```python
from build123d import *

# Parameters (mm, degrees)
F1_DEPTH = 63.5
F0_W     = 25.4
F0_H     = 16.5099985898
F2_DEPTH = 25.4
F3_DEPTH = 8.255


with BuildPart() as f1:
    # F0 (on Front) → F1 (new body, symmetric)
    with BuildSketch(Plane.XZ):
        Polygon((24.7650014102, 9.525), (-41.275, 9.525), (-41.275, -9.525), (41.275, -9.525), (41.275, 9.525), align=None)
    extrude(amount=F1_DEPTH, both=True)

    # F0 (on Front) → F2 (join, symmetric)
    with BuildSketch(Plane.XZ):
        with BuildLine():
            Line((24.7650014102, 27.0002), (24.7650014102, 9.525))
            Line((24.7650014102, 9.525), (41.275, 9.525))
            Line((41.275, 9.525), (41.275, 27.0002))
            ThreePointArc((41.275, 27.0002), (45.9246798487, 38.2255201513), (57.15, 42.8752))
            Line((57.15, 42.8752), (60.325, 42.8752))
            Line((60.325, 42.8752), (60.325, 59.3851985898))
            Line((60.325, 59.3851985898), (57.15, 59.3851985898))
            add(Edge.make_bspline(
                [(56.1071182256, 59.3684024719), (56.4564666589, 59.3745204877), (56.8041138662, 59.3801120386), (57.15, 59.3851985898)],
                knots=[109.340800828, 109.340800828, 109.340800828, 109.340800828, 110.3336758583, 110.3336758583, 110.3336758583, 110.3336758583], degree=3))
            ThreePointArc((56.1071182256, 59.3684024719), (33.8845550392, 49.5281205528), (24.7650014102, 27.0002))
        make_face()
        with Locations((73.025, 51.1301992949)):
            Rectangle(F0_W, F0_H)
    extrude(amount=F2_DEPTH, both=True)

    # F0 (on Front) → F3 (join, symmetric)
    with BuildSketch(Plane.XZ):
        with BuildLine():
            add(Edge.make_bspline(
                [(-41.275, 9.525), (-41.4689933248, 51.6361419003), (17.6349678521, 58.6946532825), (56.1071182256, 59.3684024719)],
                knots=[0, 0, 0, 0, 109.340800828, 109.340800828, 109.340800828, 109.340800828], degree=3))
            Line((-41.275, 9.525), (24.7650014102, 9.525))
            Line((24.7650014102, 9.525), (24.7650014102, 27.0002))
            ThreePointArc((24.7650014102, 27.0002), (33.8845550392, 49.5281205528), (56.1071182256, 59.3684024719))
        make_face()
    extrude(amount=F3_DEPTH, both=True)

    # F0 (on Front) → F4 (revolve)
    with BuildSketch(Plane.XZ):
        Polygon((85.725, 66.675), (85.725, 59.3851985898), (85.725, 42.8752), (85.725, 38.1), (111.125, 38.1), (111.125, 66.675), align=None)
    revolve(axis=Axis((85.725, 0, 52.3875), (0, 0, 1)))


solid = f1.part
```
For this review, take the finished solid that the model builds, in its own axes (mm). A direction names the side the tool comes from. Give positions to 0.01 mm unless a question says otherwise; leave off trailing zeros. Loops run counter-clockwise (first coordinate to the right, second up) from the corner with the lowest first, then second, coordinate; pieces in that order, holes last. Notation, with made-up numbers: M 78.5,61 L 87.5,61 A32 ccw 87.5,97 Z; hole C 19,39.5 d3. An arc over 180 degrees is marked long. One line per item, written item: value. Start each with the question number.
Q1. Add section B-B (z = 3). Give the boundary of the cut face in (x, y) (3 decimals).
Q2. Machinability: for faces 1 (the face through (60, -2, 59.385)), 2 (the face through (34.13, -16.95, 49.78)), 3 (the face through (-3, 8.255, 29)), 4 (the face through (48, 25.4, 40.3)), which of the approach directions +Z, -Z, +X, -X, +Y, -Y give a long, thin tool a straight path to every point of the face, cutting with its end or side? Answer none if there is none.
Q3. For L1, parallel to Z at x = -25.5, y = 29 (3 decimals); L2, parallel to Y at x = 43.5, z = 47; L3, parallel to Y at x = -10, z = 40 (3 decimals), list the stretches that pass through material, from the lowest coordinate up.
Q4. Add section C-C (y = -39.5). Give the boundary of the cut face in (x, z) (3 decimals), and give its area (3 significant figures).
Q5. Add section A-A (x = 71.5). Give the boundary of the cut face in (y, z) (3 decimals).
Q6. Draft analysis for pull direction X (two halves, no side actions). For faces 5 (the face through (34.13, 16.71, 49.78)), 6 (the face through (86, 0, 38.1)), 7 (the face through (60, 2, 42.875)), 8 (the face through (45.8, -0.4, 38.1)), state which applies: released by +X, released by -X, zero draft, split by the parting line, or undercut.
Q7. Clearance check with flat-ended pins moving along their axes: pin 1 Ø8.5 at (y, z) = (-21, 18.5) entering from -X (3 decimals); pin 2 Ø1 at (y, z) = (3.5, 23) entering from +X (3 decimals); pin 3 Ø23 at (x, y) = (73.5, 6.5) entering from -Z. State where each tip first meets the part, or that it passes through.
Reply:
1. outline: M -41.275,-63.5 L 41.275,-63.5 L 41.275,63.5 L -41.275,63.5 Z
2. face 1: +Z, -X
2. face 2: +Z, -X, -Y
2. face 3: +Z, -X, +Y
2. face 4: +Z, +X, -X, +Y
3. L1: -9.525 to 9.525
3. L2: -25.4 to 25.4
3. L3: -8.255 to 8.255
4. outline: M -41.275,-9.525 L 41.275,-9.525 L 41.275,9.525 L -41.275,9.525 Z
4. area: 1,570 mm²
5. outline: M -25.4,42.875 L -21.043,42.875 L -21.043,38.1 L 21.043,38.1 L 21.043,42.875 L 25.4,42.875 L 25.4,59.385 L 21.043,59.385 L 21.043,66.675 L -21.043,66.675 L -21.043,59.385 L -25.4,59.385 Z
6. face 5: released by -X
6. face 6: zero draft
6. face 7: undercut
6. face 8: undercut
7. pin 1: x = 24.765
7. pin 2: x = 41.275
7. pin 3: z = 38.1
